```python
from build123d import *

# Parameters (mm, degrees)
F0_W      = 177.8
F0_H      = 152.4
F1_DEPTH  = 53.975
F2_W      = 44.4769412279
F2_H      = 42.7047908306
F3_DEPTH  = 57.28848
F4_R      = 5.08
F5_DEPTH  = 25.4
F7_DEPTH  = 53.071
F8_R      = 18.7092621325
F9_DEPTH  = 76.2
F11_D     = 25.4
F11_DEPTH = 101.6
F11_TIP   = 7.6309298617
F12_R     = 32.2387341202
F13_DEPTH = 12.41914
F14_R     = 5.08
F15_DEPTH = 0.30507
F16_DEPTH = 1.0725


with BuildPart() as f1:
    # F0 (on Top) → F1 (new body)
    with BuildSketch(Plane.XY):
        with Locations((132.4584333658, -75.6843322992)):
            Rectangle(F0_W, F0_H)
    extrude(amount=F1_DEPTH)

    # F2 (on face) → F3 (cut)
    with BuildSketch(Plane.XY.offset(53.975)):
        with Locations((199.1199627519, -130.5319368839)):
            Rectangle(F2_W, F2_H)
    extrude(amount=-F3_DEPTH, mode=Mode.SUBTRACT)

    # F4
    f4_edges = [f1.edges().sort_by_distance(p)[0] for p in [
        (176.881492, -130.531937, 53.975),
        (110.219963, -151.884332, 53.975),
    ]]
    fillet(f4_edges, radius=F4_R)

    # F5 (cut): a face of the model
    f5_faces = [f1.faces().sort_by_distance(p)[0] for p in [
        (221.3584333658, -54.3319368839, 26.9875),
    ]]
    extrude(f5_faces, amount=-F5_DEPTH, mode=Mode.SUBTRACT)

    # F6 (on face) → F7 (join)
    with BuildSketch(Plane.XY.offset(53.975)):
        Polygon((195.9584333658, 0.5156677008), (195.9584333658, -109.1795414686), (239.5593672991, -11.6872834042), (245.01273036, -0.1214179429), (236.9844764471, 0.5156677008), align=None)
    extrude(amount=-F7_DEPTH)

    # F8 (on face) → F9 (join)
    with BuildSketch(Plane.XY.offset(53.975)):
        with Locations((90.3183594346, -53.666587919)):
            Circle(F8_R)
    extrude(amount=F9_DEPTH)

    # F11
    with Locations(Plane.XY.offset(130.175)):
        with Locations((90.3183594346, -53.666587919)):
            Hole(F11_D / 2, depth=F11_DEPTH)
            with Locations((0, 0, -(F11_DEPTH + F11_TIP / 2))):  # 118° drill point
                Cone(0, F11_D / 2, F11_TIP, mode=Mode.SUBTRACT)

    # F12 (on face) → F13 (join)
    with BuildSketch(Plane.XY.offset(53.975)):
        with Locations((90.3183594346, -53.666587919)):
            Circle(F12_R)
    extrude(amount=F13_DEPTH)

    # F14
    f14_edges = [f1.edges().sort_by_distance(p)[0] for p in [
        (58.079625, -53.666588, 66.39414),
        (71.609097, -53.666588, 66.39414),
    ]]
    fillet(f14_edges, radius=F14_R)

    # F15 (add): faces of the model
    f15_faces = [f1.faces().sort_by_distance(p)[0] for p in [
        (212.3023430426, -36.0634157102, 0.904),
        (117.3351859078, -73.6905388833, 0),
    ]]
    extrude(f15_faces, amount=F15_DEPTH)

    # F16 (add): a face of the model
    f16_faces = [f1.faces().sort_by_distance(p)[0] for p in [
        (212.3023430426, -36.0634157102, 0.59893),
    ]]
    extrude(f16_faces, amount=F16_DEPTH)


solid = f1.part
```
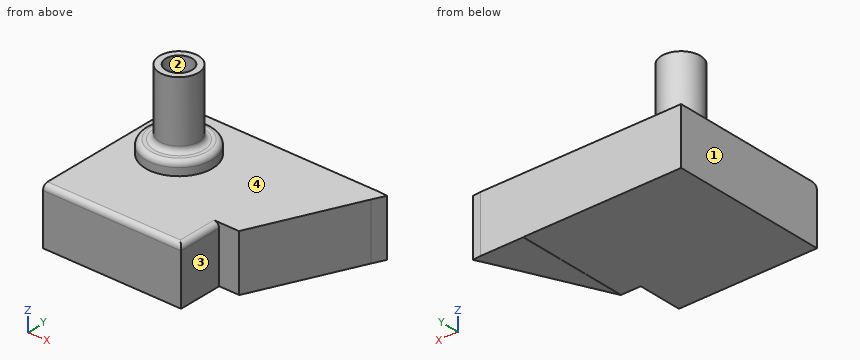
Geometry check sheet. Reference: the model listing, model coordinates, mm. Face numbers are marked on the shaded views. Coordinates: 2 decimals unless noted, no trailing zeros. Loops run counter-clockwise (first coordinate to the right, second up) from the corner with the lowest first, then second, coordinate; pieces in that order, holes last. Notation, with made-up numbers: (69, 56.5) - (127, 56.5) arc R25 ccw to (127, 86.5) - close; hole circle Ø4 at (8, -8.75). An arc over 180 degrees is marked (long way). One line per item, written item: value. Start each with the question number.
(1) Depth check by flat-ended pin: P1, Ø2, axis at x = 126.5, y = -21.5, coming from the -Z side; P2, Ø4, axis at y = -87.5, z = 34.5, coming from the +X side; P3, Ø7, axis at x = 183, z = 16.5, coming from the -Y side. Enter the tip coordinate at first touch or a pass-through.
(2) Material ranges on line 1 (Z direction, x = 186, y = -70) (3 decimals); line 2 (Y direction, x = 86.5, z = 74); line 3 (X direction, y = -59, z = 67), recorded low to high. Write a range as [from, to].
(3) Cross-section at B-B on y = -123. Enter the section's corners in (x, z) (1 decimal), plus the area to 3 significant figures.
(4) Cross-section at A-A on z = 37. Enter the section's corners in (x, y), plus the area to 3 significant figures.
(5) Mould release check, pull along X, two halves, no side actions. Record for the marked faces 1, 2, 3 and 4: released by +X, released by -X, zero draft, split by the parting line, or undercut.
(6) Cross-section at D-D on x = 157.5. Enter the section's corners in (y, z) (3 decimals).
(7) Cross-section at C-C on z = 9. Enter the section's corners in (x, y), plus the area to 3 significant figures.
Results below:
1. P1: stops at z = -0.31
1. P2: stops at x = 206.55
1. P3: stops at y = -109.18
2. line 1: z = [-0.305, 53.975]
2. line 2: y = [-71.98, -65.78], [-41.55, -35.35]
2. line 3: x = [69.61, 78.79], [101.84, 111.03]
3. outline: (43.6, -0.3) - (176.9, -0.3) - (176.9, 48.9) arc R5.1 ccw to (171.8, 54) - (43.6, 54) - close
3. area: 7,230 mm2
4. outline: (43.56, -151.88) - (176.88, -151.88) - (176.88, -109.18) - (195.96, -109.18) - (239.56, -11.69) - (245.01, -0.12) - (236.98, 0.52) - (43.56, 0.52) - close; hole circle Ø25.4 at (90.32, -53.67)
4. area: 24,600 mm2
5. face 1: released by -X
5. face 2: undercut
5. face 3: released by +X
5. face 4: zero draft
6. outline: (-151.884, -0.305) - (0.516, -0.305) - (0.516, 53.975) - (-146.804, 53.975) arc R5.08 ccw to (-151.884, 48.895) - close
7. outline: (43.56, -151.88) - (176.88, -151.88) - (176.88, -109.18) - (195.96, -109.18) - (239.56, -11.69) - (245.01, -0.12) - (236.98, 0.52) - (43.56, 0.52) - close
7. area: 25,100 mm2
